```python
from build123d import *

# Parameters (mm, degrees)
BOSS_EXTRUDE1_DEPTH = 5
SKETCH2_R           = 1.5
CUT_EXTRUDE1_DEPTH  = 5
CIRPATTERN1_COUNT   = 4
CIRPATTERN1_ANGLE   = 168
SKETCH8_W           = 25
SKETCH8_H           = 10
CUT_EXTRUDE3_DEPTH  = 5
SKETCH9_W           = 120
SKETCH9_H           = 20
BOSS_EXTRUDE5_DEPTH = 5
SKETCH10_R          = 5
CUT_EXTRUDE4_DEPTH  = 10
CHAMFER1_SIZE       = 1
CHAMFER2_SIZE       = 1
SKETCH5_R           = 1.6
CUT_EXTRUDE5_DEPTH  = 10
BOSS_EXTRUDE6_START = 1
SKETCH11_R          = 2.5
SKETCH11_R_2        = 1.6
BOSS_EXTRUDE6_DEPTH = 1
FILLET5_R           = 1


with BuildPart() as part:
    # Sketch1 → Boss-Extrude1 (new body)
    with BuildSketch(Plane(origin=(0, 0, 0), x_dir=(1, 0, 0), z_dir=(0, 1, 0))):
        with BuildLine():
            Line((-60, 0), (-25.75, 0))
            Line((-25.75, 0), (25.75, 0))
            Line((25.75, 0), (60, 0))
            ThreePointArc((60, 0), (0, 60), (-60, 0))
        make_face()
    extrude(amount=BOSS_EXTRUDE1_DEPTH)

    # Sketch2 → Cut-Extrude1 (cut)
    with BuildSketch(Plane(origin=(0, 5, 0), x_dir=(1, 0, 0), z_dir=(0, 1, 0))):
        with Locations(Location((-54.772255751, 5, 0), (0, 0, 270))):
            Circle(SKETCH2_R)
    cut_extrude1 = extrude(amount=-CUT_EXTRUDE1_DEPTH, mode=Mode.SUBTRACT)

    # CirPattern1: Cut-Extrude1 ×4 about axis
    cirpattern1_axis = Axis((0, 0, 0), (0, -1, 0))
    for i in range(1, CIRPATTERN1_COUNT):
        add(cut_extrude1.rotate(cirpattern1_axis, i * CIRPATTERN1_ANGLE / (CIRPATTERN1_COUNT - 1)), mode=Mode.SUBTRACT)

    # Sketch8 → Cut-Extrude3 (cut, symmetric)
    with BuildSketch(Plane(origin=(0, 0, 0), x_dir=(-1, 0, 0), z_dir=(0, -1, 0))):
        with Locations((0, 15)):
            Rectangle(SKETCH8_W, SKETCH8_H)
    extrude(amount=CUT_EXTRUDE3_DEPTH, both=True, mode=Mode.SUBTRACT)

    # Sketch9 → Boss-Extrude5 (add)
    with BuildSketch(Plane.XY):
        with Locations((0, -5)):
            Rectangle(SKETCH9_W, SKETCH9_H)
    extrude(amount=BOSS_EXTRUDE5_DEPTH)

    # Sketch10 → Cut-Extrude4 (cut)
    with BuildSketch(Plane(origin=(0, 5, 0), x_dir=(1, 0, 0), z_dir=(0, 1, 0))):
        with Locations(Location((0, 40, 0), (0, 0, 270))):
            Circle(SKETCH10_R)
    extrude(amount=-CUT_EXTRUDE4_DEPTH, mode=Mode.SUBTRACT)

    # Chamfer1
    chamfer1_edges = [part.edges().sort_by_distance(p)[0] for p in [
        (-54.772255751, 5, -6.5),
        (-25.239512501, 5, -49.043011823),
        (26.544743195, 5, -48.349008353),
        (54.926776539, 5, -5.029832898),
        (-12.5, 5, -15),
        (0, 5, -10),
        (12.5, 5, -15),
        (0, 5, -20),
        (0, 5, -45),
    ]]
    chamfer(chamfer1_edges, length=CHAMFER1_SIZE)

    # Chamfer2
    chamfer2_edges = [part.edges().sort_by_distance(p)[0] for p in [
        (0, 5, -60),
        (-60, 5, 2.5),
        (60, 5, 2.5),
        (0, 5, 5),
    ]]
    chamfer(chamfer2_edges, length=CHAMFER2_SIZE)

    # Sketch5 → Cut-Extrude5 (cut)
    with BuildSketch(Plane.XZ):
        with Locations(Location((-7.785, -26.572067281, 0), (0, 0, 270))):
            Circle(SKETCH5_R)
        with Locations(Location((7.775, -26.572067281, 0), (0, 0, 270))):
            Circle(SKETCH5_R)
    extrude(amount=-CUT_EXTRUDE5_DEPTH, mode=Mode.SUBTRACT)

    # Sketch11 → Boss-Extrude6 (add)
    # profile 1 of 2: a face of its own
    with BuildSketch(Plane.XZ.offset(BOSS_EXTRUDE6_START)):
        with Locations(Location((-7.785, -26.572067281, 0), (0, 0, 90))):
            Circle(SKETCH11_R)
        with Locations(Location((-7.785, -26.572067281, 0), (0, 0, 270))):
            Circle(SKETCH11_R_2, mode=Mode.SUBTRACT)
    # profile 2 of 2: a face of its own
    with BuildSketch(Plane.XZ.offset(BOSS_EXTRUDE6_START)):
        with Locations(Location((7.775, -26.572067281, 0), (0, 0, 90))):
            Circle(SKETCH11_R)
        with Locations(Location((7.775, -26.572067281, 0), (0, 0, 270))):
            Circle(SKETCH11_R_2, mode=Mode.SUBTRACT)
    extrude(amount=-BOSS_EXTRUDE6_DEPTH)

    # Fillet5
    fillet5_edges = [part.edges().sort_by_distance(p)[0] for p in [
        (-7.785, 0, -29.072067281),
        (7.775, 0, -29.072067281),
    ]]
    fillet(fillet5_edges, radius=FILLET5_R - 0.0001)  # a hair under: the kernel refuses the full size


solid = part.part
```
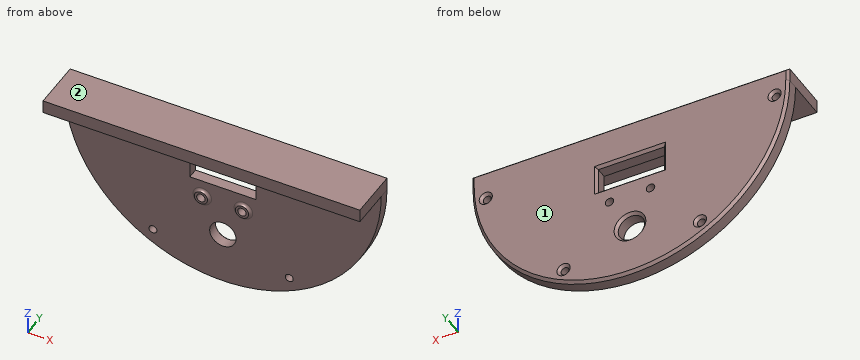
Can you work these out from the model? Positions are in its coordinate system, mm. Face numbers are marked on the shaded views. Round coordinates to 2 decimals unless told otherwise and drop trailing zeros. Order: outer loops, then holes, each group sorted by start corner. A loop starts at its lowest first (then second) coordinate and runs counter-clockwise, first axis right, second up.
(1) We'd pull the mould along Z, two halves only. Please class the marked faces 1 and 2: +Z half, -Z half, draft (parallel to the pull), parting line (faces both ways), or undercut.
Results are:
face 1: draft
face 2: +Z half
(2) If I drill on L1, parallel to X at y = 0.5, z = -27.5; L2, parallel to Y at x = 8, z = -35, over which ranges is the centre line in solid material (lowest first)?
Results are:
L1: x = -53.33 to -9.09, -6.48 to 6.47, 9.08 to 53.33
L2: y = 0 to 5
(3) If we section it at B-B (y = -5): Please give me the cut outline in (x, z).
Results are:
outline: (-60, 0) - (60, 0) - (60, 5) - (-60, 5) - close
(4) If we section it at A-A (x = 0): Please give me the cut outline in (y, z).
Results are:
outline: (-15, 0) - (0, 0) - (0, -10) - (4, -10) - (5, -9) - (5, 4) - (4, 5) - (-15, 5) - close; (0, -60) - (4, -60) - (5, -59) - (5, -46) - (4, -45) - (0, -45) - close; (0, -35) - (4, -35) - (5, -34) - (5, -21) - (4, -20) - (0, -20) - close
(5) I'm going to push flat-ended pins straight in: pin 1 (8 mm diameter, centred on x = -6, y = -1, fed in from -Z); pin 2 (1.5 mm diameter, centred on x = -47, z = -37.5, fed in from +Y); pin 3 (2 mm diameter, centred on x = -19.5, z = -14, fed in from -Y). Where does each tip first touch, or does it pass through?
Results are:
pin 1: stops at z = -59.96
pin 2: stops at y = 4.62
pin 3: stops at y = 0
